Verification items for this drawing (mm, ordinates from the low corner). Round coordinates to 2 decimals unless told otherwise and drop trailing zeros. Loops run counter-clockwise (first coordinate to the right, second up) from the corner with the lowest first, then second, coordinate; pieces in that order, holes last. Notation, with made-up numbers: (-40, 9) - (-2, 9) arc R12 cw to (-2, 27) - close; hole circle Ø1 at (-20, -2.75). An arc over 180 degrees is marked (long way). Put each result on its own line as item: value.
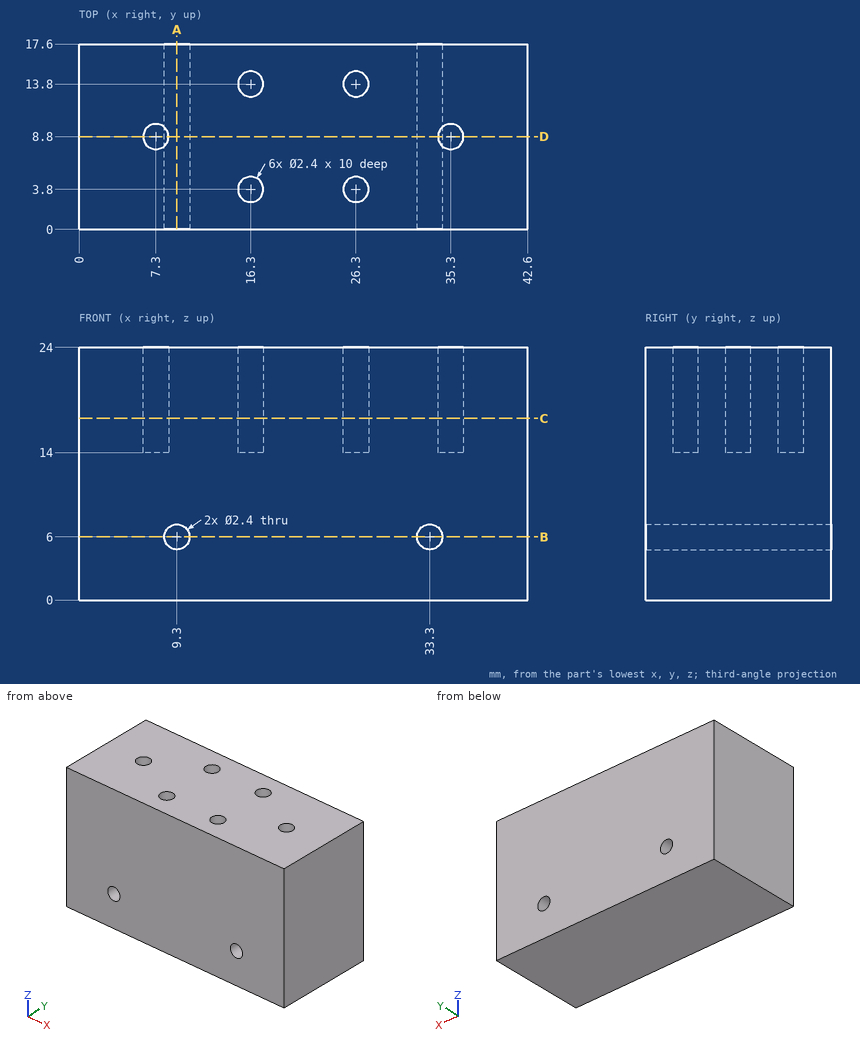
Item 1: Section check B-B on z = 6. Enter the section's corners in (x, y), then the cut area to 3 significant figures.
Filled sheet:
outline: (0, 0) - (8.1, 0) - (8.1, 17.6) - (0, 17.6) - close; (10.5, 0) - (32.1, 0) - (32.1, 17.6) - (10.5, 17.6) - close; (34.5, 0) - (42.6, 0) - (42.6, 17.6) - (34.5, 17.6) - close
area: 665 mm²
Item 2: Thickness scan on line 1 (X direction, y = 6.75, z = 6); line 2 (Y direction, x = 26.3, z = 18.25); line 3 (Y direction, x = 15.5, z = 14.25). Record the ranges inside material, lowest first. Write a range as from..to.
Filled sheet:
line 1: 0..8.1, 10.5..32.1, 34.5..42.6
line 2: 0..2.6, 5..12.6, 15..17.6
line 3: 0..2.91, 4.69..12.91, 14.69..17.6
Item 3: Section check A-A on x = 9.3. Enter the section's corners in (y, z).
Filled sheet:
outline: (0, 0) - (17.6, 0) - (17.6, 4.8) - (0, 4.8) - close; (0, 7.2) - (17.6, 7.2) - (17.6, 24) - (0, 24) - close
Item 4: Section check D-D on y = 8.8. Enter the section's corners in (x, z).
Filled sheet:
outline: (0, 0) - (42.6, 0) - (42.6, 24) - (36.5, 24) - (36.5, 14) - (34.1, 14) - (34.1, 24) - (8.5, 24) - (8.5, 14) - (6.1, 14) - (6.1, 24) - (0, 24) - close; hole circle Ø2.4 at (9.3, 6); hole circle Ø2.4 at (33.3, 6)
Item 5: Section check C-C on z = 17.25. Enter the section's corners in (x, y), then the cut area to 3 significant figures.
Filled sheet:
outline: (0, 0) - (42.6, 0) - (42.6, 17.6) - (0, 17.6) - close; hole circle Ø2.4 at (7.3, 8.8); hole circle Ø2.4 at (16.3, 3.8); hole circle Ø2.4 at (16.3, 13.8); hole circle Ø2.4 at (26.3, 3.8); hole circle Ø2.4 at (26.3, 13.8); hole circle Ø2.4 at (35.3, 8.8)
area: 723 mm²
